The model under review builds one solid part; all positions refer to its coordinate system, in mm. A direction names the side the tool comes from. Give positions to 0.01 mm unless a question says otherwise; leave off trailing zeros. Order: outer loops, then holes, each group sorted by start corner. A loop starts at its lowest first (then second) coordinate and runs counter-clockwise, first axis right, second up. Notation, with made-up numbers: (-31.5, -25.75) - (-8.5, -25.75) arc R19 cw to (-8.5, -14.75) - close; hole circle Ø2 at (-5, 13.25). An arc over 180 degrees is marked (long way). Answer as CSV lines item,"result". Start each with the question number.
from build123d import *

# Parameters (mm, degrees)
F1_DEPTH = 1
F2_D     = 4
F3_D     = 2


with BuildPart() as f1:
    # F0 (on Top) → F1 (new body)
    with BuildSketch(Plane.XY):
        with BuildLine():
            Line((20, 12), (20, 20))
            Line((20, 20), (12, 20))
            Line((12, 20), (8, 20))
            Line((8, 20), (-8, 20))
            ThreePointArc((-8, 20), (-10, 18), (-12, 20))
            Line((-12, 20), (-20, 20))
            Line((-20, 20), (-20, 12))
            Line((-20, 12), (-20, 8))
            Line((-20, 8), (-20, -8))
            ThreePointArc((-20, -8), (-18.5857864376, -8.5857864376), (-18, -10))
            ThreePointArc((-18, -10), (-18.5857864376, -11.4142135624), (-20, -12))
            Line((-20, -12), (-20, -20))
            Line((-20, -20), (-12, -20))
            Line((-12, -20), (-8, -20))
            Line((-8, -20), (8, -20))
            ThreePointArc((8, -20), (10, -18), (12, -20))
            Line((12, -20), (20, -20))
            Line((20, -20), (20, -12))
            Line((20, -12), (20, -8))
            Line((20, -8), (20, 8))
            ThreePointArc((20, 8), (18, 10), (20, 12))
        make_face()
        with BuildLine():
            Line((8, 20), (12, 20))
            ThreePointArc((12, 20), (10, 22), (8, 20))
        make_face()
        with BuildLine():
            ThreePointArc((22, 10), (21.4142135624, 11.4142135624), (20, 12))
            Line((20, 12), (20, 8))
            ThreePointArc((20, 8), (21.4142135624, 8.5857864376), (22, 10))
        make_face()
        with BuildLine():
            Line((20, 8), (20, 12))
            ThreePointArc((20, 12), (18, 10), (20, 8))
        make_face()
        with BuildLine():
            ThreePointArc((-12, 20), (-10, 18), (-8, 20))
            Line((-8, 20), (-12, 20))
        make_face()
        with BuildLine():
            Line((-12, 20), (-8, 20))
            ThreePointArc((-8, 20), (-10, 22), (-12, 20))
        make_face()
        with BuildLine():
            ThreePointArc((20, -12), (22, -10), (20, -8))
            Line((20, -8), (20, -12))
        make_face()
        with BuildLine():
            Line((-20, 8), (-20, 12))
            ThreePointArc((-20, 12), (-22, 10), (-20, 8))
        make_face()
        with BuildLine():
            ThreePointArc((8, -20), (10, -22), (12, -20))
            Line((12, -20), (8, -20))
        make_face()
        with BuildLine():
            Line((8, -20), (12, -20))
            ThreePointArc((12, -20), (10, -18), (8, -20))
        make_face()
        with BuildLine():
            ThreePointArc((-18, -10), (-18.5857864376, -8.5857864376), (-20, -8))
            Line((-20, -8), (-20, -12))
            ThreePointArc((-20, -12), (-18.5857864376, -11.4142135624), (-18, -10))
        make_face()
        with BuildLine():
            Line((-20, -12), (-20, -8))
            ThreePointArc((-20, -8), (-22, -10), (-20, -12))
        make_face()
        with BuildLine():
            ThreePointArc((-12, -20), (-10, -22), (-8, -20))
            Line((-8, -20), (-12, -20))
        make_face()
    extrude(amount=F1_DEPTH)

    # F2 (through all)
    with Locations(Plane(origin=(0, 0, 0), x_dir=(1, 0, 0), z_dir=(0, 0, -1))):
        with Locations((-20, 10), (-10, -20), (20, -10), (10, 20)):
            Hole(F2_D / 2)

    # F3 (through all)
    with Locations(Plane(origin=(0, 0, 0), x_dir=(1, 0, 0), z_dir=(0, 0, -1))):
        with Locations((10, -20), (-20, -10), (-10, 20), (20, 10)):
            Hole(F3_D / 2)


solid = f1.part
Item 1: For line 1 along X through (y, z) = (10, 0.65); line 2 along X through (y, z) = (-10, 0.45), list the stretches that pass through material, from the lowest coordinate up.
Item 2: Machinability: for faces 1 (the face through (-10, 18, 0.5)), 2 (the face through (-20, 16.1, 0.5)), 3 (the face through (-0.1, -20, 0.5)), 4 (the face through (20, 15.9, 0.5)), 5 (the face through (-16.1, -20, 0.5)), which of the approach directions +Z, -Z, +X, -X, +Y, -Y give a long, thin tool a straight path to every point of the face, cutting with its end or side? Answer none if there is none.
Item 3: Take a section at B-B on z = 0.15. Write out the cut boundary in (x, y).
Item 4: Clearance check with flat-ended pins moving along their axes: pin 1 (1.8 mm diameter, centred on x = -20, y = 10, fed in from +Z); pin 2 (0.5 mm diameter, centred on y = 16, z = 0.5, fed in from -X). State where each tip first meets the part, or that it passes through.
Item 5: Mouldability with a two-part tool opening along Y and no side actions: class faces 6 (the face through (0.1, 20, 0.5)), 7 (the face through (-20, -15.9, 0.5)), 8 (the face through (-18, -10, 0.5)) as released by +Y, released by -Y, zero draft, split by the parting line, or undercut.
Item 6: Take a section at A-A on y = 10. Write out the cut boundary in (x, z).
Item 7: Take a section at D-D on x = 14.5. Write out the cut boundary in (y, z).
Data:
1,line 1,"x = -22 to -21, -19 to 18"
1,line 2,"x = -18 to 19, 21 to 22"
2,face 1,"+Z, -Z, +Y"
2,face 2,"+Z, -Z, -X, +Y"
2,face 3,"+Z, -Z, +X, -Y"
2,face 4,"+Z, -Z, +X, +Y"
2,face 5,"+Z, -Z, -X, -Y"
3,outline,"(-20, -20) - (-12, -20) arc R2 ccw to (-8, -20) - (8, -20) arc R2 cw to (12, -20) - (20, -20) - (20, -12) arc R2 ccw to (20, -8) - (20, 8) arc R2 cw to (20, 12) - (20, 20) - (12, 20) arc R2 ccw to (8, 20) - (-8, 20) arc R2 cw to (-12, 20) - (-20, 20) - (-20, 12) arc R2 ccw to (-20, 8) - (-20, -8) arc R2 cw to (-20, -12) - close; hole circle Ø2 at (-20, 10); hole circle Ø2 at (-10, -20); hole circle Ø2 at (10, 20); hole circle Ø2 at (20, -10)"
4,pin 1,"passes through"
4,pin 2,"stops at x = -20"
5,face 6,"released by +Y"
5,face 7,"zero draft"
5,face 8,"undercut"
6,outline,"(-22, 0) - (-21, 0) - (-21, 1) - (-22, 1) - close; (-19, 0) - (18, 0) - (18, 1) - (-19, 1) - close"
7,outline,"(-20, 0) - (20, 0) - (20, 1) - (-20, 1) - close"
